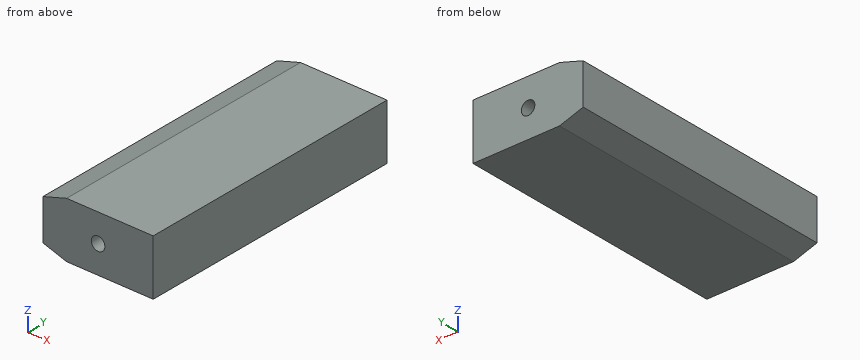
from build123d import *

# Parameters (mm, degrees)
BOSS_EXTRUDE1_DEPTH = 40
CUT_EXTRUDE1_DEPTH  = 44.965099795


with BuildPart() as part:
    # Sketch1 → Boss-Extrude1 (new body)
    with BuildSketch(Plane(origin=(0, 0, 0), x_dir=(1, 0, 0), z_dir=(0, 1, 0))):
        Polygon((-16.3, 4.1), (0, 4.1), (0, 8.2), (-12.8, 8.2), (-16.3, 7.1), align=None)
        Polygon((-12.8, 0), (0, 0), (0, 4.1), (-16.3, 4.1), (-16.3, 1.1), align=None)
    extrude(amount=BOSS_EXTRUDE1_DEPTH)

    # Sketch2 → Cut-Extrude1 (cut, through all)
    with BuildSketch(Plane(origin=(0, 40, 0), x_dir=(1, 0, 0), z_dir=(0, 1, 0))):
        with BuildLine():
            ThreePointArc((-9.15, 4.1), (-8.15, 3.1), (-7.15, 4.1))
            Line((-7.15, 4.1), (-9.15, 4.1))
        make_face()
        with BuildLine():
            Line((-9.15, 4.1), (-7.15, 4.1))
            ThreePointArc((-7.15, 4.1), (-8.15, 5.1), (-9.15, 4.1))
        make_face()
    extrude(amount=-CUT_EXTRUDE1_DEPTH, mode=Mode.SUBTRACT)


solid = part.part
Verification items for the finished model (mm, model axes). Give positions to 0.01 mm unless a question says otherwise; leave off trailing zeros. Loops run counter-clockwise (first coordinate to the right, second up) from the corner with the lowest first, then second, coordinate; pieces in that order, holes last.
1) Sectioned sample at A-A, the plane z = -4.1. Enter the section's corners in (x, y).
2) Sectioned sample at B-B, the plane x = -8.15. Enter the section's corners in (y, z), then the cut area to 3 significant figures.
3) Sectioned sample at D-D, the plane z = -7.5. Enter the section's corners in (x, y).
4) Thickness scan on line 1 along X through (y, z) = (30.5, -4.1); line 2 along Z through (x, y) = (-8.15, 32.5); line 3 along X through (y, z) = (18, -5). Record the ranges inside material, lowest first.
5) Sectioned sample at C-C, the plane y = 19. Enter the section's corners in (x, z), then the cut area to 3 significant figures.
6) Depth check by flat-ended pin: pin 1 Ø3 at (x, z) = (-2, -7.5) entering from -Y. Enter the tip coordinate at first touch or a pass-through.
Answers:
1. outline: (-16.3, 0) - (-9.15, 0) - (-9.15, 40) - (-16.3, 40) - close; (-7.15, 0) - (0, 0) - (0, 40) - (-7.15, 40) - close
2. outline: (0, -8.2) - (40, -8.2) - (40, -5.1) - (0, -5.1) - close; (0, -3.1) - (40, -3.1) - (40, 0) - (0, 0) - close
2. area: 248 mm2
3. outline: (-15.03, 0) - (0, 0) - (0, 40) - (-15.03, 40) - close
4. line 1: x = -16.3 to -9.15, -7.15 to 0
4. line 2: z = -8.2 to -5.1, -3.1 to 0
4. line 3: x = -16.3 to -8.59, -7.71 to 0
5. outline: (-16.3, -7.1) - (-12.8, -8.2) - (0, -8.2) - (0, 0) - (-12.8, 0) - (-16.3, -1.1) - close; hole circle Ø2 at (-8.15, -4.1)
5. area: 127 mm2
6. pin 1: stops at y = 0
